Build history of the part. All positions in model axes, mm. Face numbers are marked on the shaded views. A direction names the side the tool comes from. Round coordinates to 2 decimals unless told otherwise and drop trailing zeros. Order: outer loops, then holes, each group sorted by start corner. A loop starts at its lowest first (then second) coordinate and runs counter-clockwise, first axis right, second up. Notation, with made-up numbers: M 49,8 L 71,8 A21 ccw 71,17 Z; hole C 27,58 d4. An arc over 180 degrees is marked long. One line per item, written item: value. Start each with the question number.
Item 1: Band-saw the part on D-D, the plane x = 12. Write the cut outline in (y, z).
Item 2: Band-saw the part on A-A, the plane x = 22.25. Write the cut outline in (y, z), then the cut area to 3 significant figures.
Item 3: Probe L1, parallel to X at y = 28.85, z = 6; L2, parallel to Y at x = 15.75, z = 2.5; L3, parallel to Y at x = 18, z = 8.25. List the from-to ranges inside material, lowest first.
Item 4: Tool access for the marked faces 5, 6 and 7: list every direction of +Z, -Z, +X, -X, +Y, -Y with a clear straight run to the whole face (end or side of a thin tool).
Item 5: Two-plate mould, pull along Y, no slides. Class the marked faces 1, 2, 3 and 4: +Y half, -Y half, draft (parallel to the pull), parting line (faces both ways), or undercut.
Item 6: Pin check, flat tips, straight feed: pin 1 (1 mm diameter, centred on x = 20.5, z = 6, fed in from -Y); pin 2 (3 mm diameter, centred on y = 2.5, z = 4, fed in from -X); pin 3 (2.5 mm diameter, centred on x = 15, z = 6, fed in from +Y); pin 4 (3 mm diameter, centred on x = 13.5, y = 25, fed in from -Z). Stop position of each tip, or through.
Item 7: Band-saw the part on B-B, the plane z = 6. Write the cut outline in (x, y), then the cut area to 3 significant figures.
Item 8: Band-saw the part on C-C, the plane y = 29.5. Write the cut outline in (x, z).
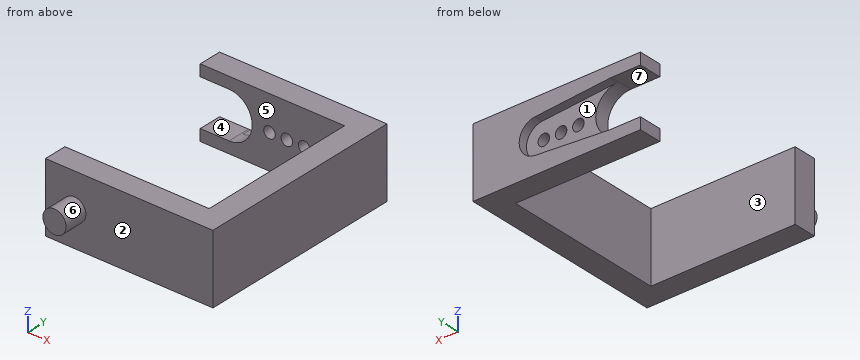
```python
from build123d import *

# Parameters (mm, degrees)
EXTRUDE_1_DEPTH     = 12
CUT_EXTRUDE_1_DEPTH = 5.1
CUT_EXTRUDE_2_DEPTH = 1.5
SKETCH_4_3_R        = 1
CUT_EXTRUDE_3_DEPTH = 6.5
SKETCH_2_R          = 2
EXTRUDE_2_DEPTH     = 4.1


with BuildPart() as part:
    # 草图1 → 凸台-拉伸1 (new body)
    with BuildSketch(Plane.XY):
        Polygon((0, 0), (25, 0), (25, 28), (0, 28), (0, 32), (29, 32), (29, -4), (0, -4), align=None)
    extrude(amount=EXTRUDE_1_DEPTH)

    # 草图3 → 切除-拉伸1 (cut)
    with BuildSketch(Plane(origin=(0, 32, 0), x_dir=(1, 0, 0), z_dir=(0, 1, 0))):
        with BuildLine():
            Line((5, -2), (0, -2))
            Line((0, -2), (0, -10))
            Line((0, -10), (5, -10))
            ThreePointArc((5, -10), (9, -6), (5, -2))
        make_face()
    extrude(amount=-CUT_EXTRUDE_1_DEPTH, mode=Mode.SUBTRACT)

    # 草图4 → 切除-拉伸2 (cut)
    with BuildSketch(Plane(origin=(0, 32, 0), x_dir=(1, 0, 0), z_dir=(0, 1, 0))):
        with BuildLine():
            Line((18.230769231, -3.008888908), (5.307692308, -2.011851878))
            ThreePointArc((5.307692308, -2.011851878), (9, -6), (5.307692308, -9.988148122))
            Line((5.307692308, -9.988148122), (18.230769231, -8.991111092))
            ThreePointArc((18.230769231, -8.991111092), (21, -6), (18.230769231, -3.008888908))
        make_face()
    extrude(amount=-CUT_EXTRUDE_2_DEPTH, mode=Mode.SUBTRACT)

    # 草图4<3> → 切除-拉伸3 (cut)
    with BuildSketch(Plane(origin=(0, 32, 0), x_dir=(1, 0, 0), z_dir=(0, 1, 0))):
        with Locations((12, -6)):
            Circle(SKETCH_4_3_R)
        with Locations((15, -6)):
            Circle(SKETCH_4_3_R)
        with Locations((18, -6)):
            Circle(SKETCH_4_3_R)
    extrude(amount=-CUT_EXTRUDE_3_DEPTH, mode=Mode.SUBTRACT)

    # 草图2 → 凸台-拉伸2 (add)
    with BuildSketch(Plane.XZ.offset(4)):
        with Locations((5, 6)):
            Circle(SKETCH_2_R)
    extrude(amount=EXTRUDE_2_DEPTH)


solid = part.part
```
Output:
1. outline: M -4,0 L 0,0 L 0,12 L -4,12 Z; M 28,0 L 32,0 L 32,2.53 L 30.5,2.53 L 30.5,5 L 28,5 Z; M 28,7 L 30.5,7 L 30.5,9.47 L 32,9.47 L 32,12 L 28,12 Z
2. outline: M -4,0 L 0,0 L 0,12 L -4,12 Z; M 28,0 L 32,0 L 32,12 L 28,12 Z
2. area: 96.0 mm²
3. L1: x = 9 to 11, 13 to 14, 16 to 17, 19 to 29
3. L2: y = -4 to 0, 28 to 32
3. L3: y = -4 to 0, 28 to 30.5
4. face 5: +Z, -Z, -X
4. face 6: -Y
4. face 7: -X, +Y
5. face 1: +Y half
5. face 2: -Y half
5. face 3: undercut
5. face 4: draft
6. pin 1: stops at y = -4
6. pin 2: stops at x = 25
6. pin 3: stops at y = 30.5
6. pin 4: passes through
7. outline: M 0,-4 L 3,-4 L 3,-8.1 L 7,-8.1 L 7,-4 L 29,-4 L 29,32 L 21,32 L 21,30.5 L 19,30.5 L 19,28 L 25,28 L 25,0 L 0,0 Z; M 9,28 L 11,28 L 11,30.5 L 9,30.5 Z; M 13,28 L 14,28 L 14,30.5 L 13,30.5 Z; M 16,28 L 17,28 L 17,30.5 L 16,30.5 Z
7. area: 291 mm²
8. outline: M 0,0 L 29,0 L 29,12 L 0,12 L 0,10 L 5,10 A4 cw 5,2 L 0,2 Z; hole C 12,6 d2; hole C 15,6 d2; hole C 18,6 d2
